from build123d import *

# Parameters (mm, degrees)
SKETCH_1_W                       = 58
SKETCH_1_H                       = 30
SM_BASE_FLANGE_2_DEPTH           = 3
SM_EDGE_FLANGE_1_STRIP_W         = 22
SM_EDGE_FLANGE_1_STRIP_H         = 3
SM_EDGE_FLANGE_1_STRIP_CUT_DEPTH = 30
SM_EDGE_FLANGE_1_DEPTH           = 30
SM_EDGE_FLANGE_2_STRIP_W         = 18
SM_EDGE_FLANGE_2_STRIP_H         = 3
SM_EDGE_FLANGE_2_STRIP_CUT_DEPTH = 30
SM_EDGE_FLANGE_2_DEPTH           = 30
FILLET_1_R                       = 3
SKETCH_14_R                      = 1.5
CUT_EXTRUDE_1_DEPTH              = 87.353922899
SKETCH_15_R                      = 1.5
CUT_EXTRUDE_2_DEPTH              = 67.219332525


# Sheet-metal steps are written as plain solids
with BuildPart() as part:
    # Sketch 1 → 基体-法兰2 (new body)
    with BuildSketch(Plane.XY):
        Rectangle(SKETCH_1_W, SKETCH_1_H)
    extrude(amount=-SM_BASE_FLANGE_2_DEPTH)

    # 边线-法兰1 strip (across the edge) → 边线-法兰1 strip cut (cut)
    with BuildSketch(Plane(origin=(-29, -15, -3), x_dir=(1, 0, 0), z_dir=(0, 1, 0))):
        with Locations((-6, -1.5)):
            Rectangle(SM_EDGE_FLANGE_1_STRIP_W, SM_EDGE_FLANGE_1_STRIP_H)
    extrude(amount=SM_EDGE_FLANGE_1_STRIP_CUT_DEPTH, mode=Mode.SUBTRACT)

    # 边线-法兰1 section (across the edge) → 边线-法兰1 (add)
    with BuildSketch(Plane(origin=(-29, -15, -3), x_dir=(1, 0, 0), z_dir=(0, 1, 0))):
        with BuildLine():
            Line((-3, 5), (-3, 53))
            Line((-3, 53), (0, 53))
            Line((0, 53), (0, 5))
            ThreePointArc((0, 5), (1.464466094, 1.464466094), (5, 0))
            Line((5, 0), (5, -3))
            ThreePointArc((5, -3), (-0.656854249, -0.656854249), (-3, 5))
        make_face()
    extrude(amount=SM_EDGE_FLANGE_1_DEPTH)

    # 边线-法兰2 strip (across the edge) → 边线-法兰2 strip cut (cut)
    with BuildSketch(Plane(origin=(29, 15, -3), x_dir=(-1, 0, 0), z_dir=(0, -1, 0))):
        with Locations((-6, -1.5)):
            Rectangle(SM_EDGE_FLANGE_2_STRIP_W, SM_EDGE_FLANGE_2_STRIP_H)
    extrude(amount=SM_EDGE_FLANGE_2_STRIP_CUT_DEPTH, mode=Mode.SUBTRACT)

    # 边线-法兰2 section (across the edge) → 边线-法兰2 (add)
    with BuildSketch(Plane(origin=(29, 15, -3), x_dir=(-1, 0, 0), z_dir=(0, -1, 0))):
        with BuildLine():
            Line((-3, 3), (-3, 53))
            Line((-3, 53), (0, 53))
            Line((0, 53), (0, 3))
            ThreePointArc((0, 3), (0.878679656, 0.878679656), (3, 0))
            Line((3, 0), (3, -3))
            ThreePointArc((3, -3), (-1.242640687, -1.242640687), (-3, 3))
        make_face()
    extrude(amount=SM_EDGE_FLANGE_2_DEPTH)

    # 圆角1
    fillet_1_edges = [part.edges().sort_by_distance(p)[0] for p in [
        (-30.5, -15, -56),
        (-30.5, 15, -56),
        (30.5, 15, -56),
        (30.5, -15, -56),
    ]]
    fillet(fillet_1_edges, radius=FILLET_1_R)

    # 草图14 → 切除-拉伸1 (cut, through all)
    with BuildSketch(Plane.ZY.offset(32)):
        with Locations((-34.25, 0)):
            Circle(SKETCH_14_R)
        with Locations((-41.25, 7)):
            Circle(SKETCH_14_R)
        with Locations((-48.25, 0)):
            Circle(SKETCH_14_R)
        with Locations((-41.25, -7)):
            Circle(SKETCH_14_R)
    extrude(amount=-CUT_EXTRUDE_1_DEPTH, mode=Mode.SUBTRACT)

    # 草图15 → 切除-拉伸2 (cut, through all)
    with BuildSketch(Plane.XY):
        with Locations((19, 9)):
            Circle(SKETCH_15_R)
        with Locations((19, -9)):
            Circle(SKETCH_15_R)
        with Locations((-19, -9)):
            Circle(SKETCH_15_R)
        with Locations((-19, 9)):
            Circle(SKETCH_15_R)
    extrude(amount=-CUT_EXTRUDE_2_DEPTH, mode=Mode.SUBTRACT)


solid = part.part
Can you work these out from the model? Positions are in its coordinate system, mm. A direction names the side the tool comes from. Round coordinates to 2 decimals unless told otherwise and drop trailing zeros. Write each loop counter-clockwise with the first axis right and the second up, starting at its lowest first coordinate (ties: lowest second). Pieces come first, ordered by that corner, then holes. Notation, with made-up numbers: M 78,16 L 133,16 A18 cw 133,48 Z; hole C -12,5.25 d5. An arc over 180 degrees is marked long. Use CSV: the item, a comma, the result in double quotes.
(1) Imagine slicing it at C-C (z = -27). Write out the boundary of the cut face in (x, y).
Check values:
outline,"M -32,-15 L -29,-15 L -29,15 L -32,15 Z; M 29,-15 L 32,-15 L 32,15 L 29,15 Z"
(2) Imagine slicing it at D-D (y = 3.5). Write out the boundary of the cut face in (x, z).
Check values:
outline,"M -32,-56 L -29,-56 L -29,-8 A5 cw -24,-3 L 26,-3 A3 cw 29,-6 L 29,-56 L 32,-56 L 32,-6 A6 ccw 26,0 L -24,0 A8 ccw -32,-8 Z"
(3) I'm going to push flat-ended pins straight in: pin 1 (2.5 mm diameter, centred on x = -19, y = 9, fed in from +Z); pin 2 (1.5 mm diameter, centred on x = -2, y = -5.5, fed in from -Z). Where does each tip first touch, or does it pass through?
Check values:
pin 1,"through"
pin 2,"z = -3"
(4) We'd pull the mould along Y, two halves only. Please class faces 1 (the cylindrical face through (-30.48, -14.14, -55.1)), 2 (the cylindrical face through (-20.5, -8.93, -1.48)), 3 (the cylindrical face through (30.48, -0.91, -35.44)), 4 (the cylindrical face through (-28, 0, -5)): +Y half, -Y half, draft (parallel to the pull), parting line (faces both ways), or undercut.
Check values:
face 1,"-Y half"
face 2,"undercut"
face 3,"undercut"
face 4,"draft"
(5) I need wall thicknesses on line 1 along Y through (x, z) = (30.85, -41.25); line 2 along X through (y, z) = (8.25, -15.5); line 3 along Z through (x, y) = (-5, -4.5). Which ranges of each line are inside material? Lowest first, please.
Check values:
line 1,"-15 to -8.5, -5.5 to 5.5, 8.5 to 15"
line 2,"-32 to -29, 29 to 32"
line 3,"-3 to 0"
(6) Imagine slicing it at A-A (z = -48.25). Write out the boundary of the cut face in (x, y).
Check values:
outline,"M -32,-15 L -29,-15 L -29,-1.5 L -32,-1.5 Z; M -32,1.5 L -29,1.5 L -29,15 L -32,15 Z; M 29,-15 L 32,-15 L 32,-1.5 L 29,-1.5 Z; M 29,1.5 L 32,1.5 L 32,15 L 29,15 Z"
(7) On a 3-axis mill with a long thin cutter (end or side, diameter ignored), from which of +Z, -Z, +X, -X, +Y, -Y can I reach the whole of each face in a straight line? I mean faces 5 (the cylindrical face through (-20.5, 9.07, -1.48)), 6 (the flat face through (29, 0, -31)). Say none if no direction works.
Check values:
face 5,"+Z, -Z"
face 6,"-Z, +Y, -Y"
(8) Imagine slicing it at B-B (x = 19). Write out the boundary of the cut face in (y, z).
Check values:
outline,"M -15,-3 L -10.5,-3 L -10.5,0 L -15,0 Z; M -7.5,-3 L 7.5,-3 L 7.5,0 L -7.5,0 Z; M 10.5,-3 L 15,-3 L 15,0 L 10.5,0 Z"
